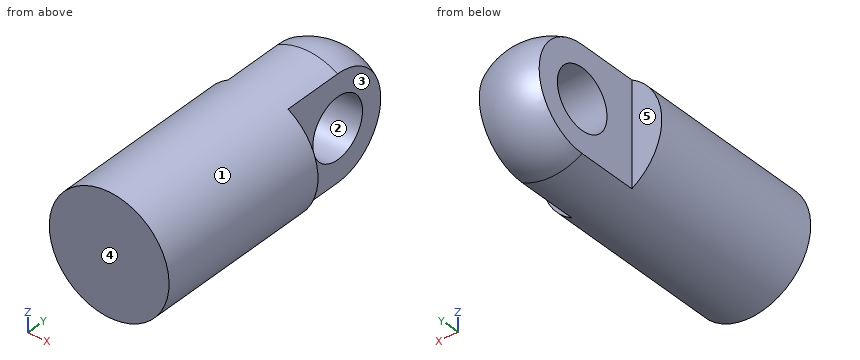
```python
from build123d import *

# Parameters (mm, degrees)
SKETCH_1_R          = 8
EXTRUDE_1_DEPTH     = 32
CUT_EXTRUDE_START   = -16
CUT_EXTRUDE_1_DEPTH = 16
SKETCH_6_R          = 4
CUT_EXTRUDE_2_DEPTH = 43.520583251


with BuildPart() as part:
    # 草图1 → 凸台-拉伸1 (new body)
    with BuildSketch(Plane(origin=(0, 0, 0), x_dir=(1, 0, 0), z_dir=(0, 1, 0))):
        with Locations(Location((0, 0, 0), (0, 0, 270))):
            Circle(SKETCH_1_R)
    extrude(amount=EXTRUDE_1_DEPTH)

    # 草图3 one side → 旋转4 (revolve)
    with BuildSketch(Plane.XY):
        with BuildLine():
            Line((0, 24), (0, 40))
            ThreePointArc((0, 40), (-8, 32), (0, 24))
        make_face()
    revolve(axis=Axis((0, 32, 0), (0, 1, 0)))

    # 草图5 → 切除-拉伸1 (cut)
    with BuildSketch(Plane(origin=(0, 40, 0), x_dir=(1, 0, 0), z_dir=(0, 1, 0)).offset(CUT_EXTRUDE_START)):
        with BuildLine():
            Line((4, -6.92820323), (4, 6.92820323))
            ThreePointArc((4, 6.92820323), (8, 0), (4, -6.92820323))
        make_face()
        with BuildLine():
            Line((-4, -6.92820323), (-4, 6.92820323))
            ThreePointArc((-4, 6.92820323), (-8, 0), (-4, -6.92820323))
        make_face()
    extrude(amount=CUT_EXTRUDE_1_DEPTH, mode=Mode.SUBTRACT)

    # 草图6 → 切除-拉伸2 (cut, through all)
    with BuildSketch(Plane(origin=(4, 0, 0), x_dir=(0, 0, -1), z_dir=(1, 0, 0))):
        with Locations((0, 32)):
            Circle(SKETCH_6_R)
    extrude(amount=-CUT_EXTRUDE_2_DEPTH, mode=Mode.SUBTRACT)


solid = part.part
```
Check sheet for the modelled part. Datum: model origin and axes. Units: mm. Face numbers are marked on the shaded views. A direction names the side the tool comes from. Round coordinates to 2 decimals unless told otherwise and drop trailing zeros. Loops run counter-clockwise (first coordinate to the right, second up) from the corner with the lowest first, then second, coordinate; pieces in that order, holes last. Notation, with made-up numbers: (-37, 68) - (-2, 68) arc R29 ccw to (-2, 100) - close; hole circle Ø6 at (16.25, 4). An arc over 180 degrees is marked (long way). Answer as a JSON object with one key per item and string values. Group by question number.
Q1. Gauge pin test, flat ends, axial feed: P1, Ø8, axis at y = 32, z = -3.5, coming from the +X side; P2, Ø1, axis at x = 2, z = -1.5, coming from the +Y side; P3, Ø1.5, axis at y = 17.5, z = 3.5, coming from the -X side; P4, Ø1.5, axis at x = 6, z = 4.5, coming from the -Y side. Record the tip position at first contact, or that the pin passes through.
Q2. Mould release check, pull along Z, two halves, no side actions. Record for the marked faces 1, 2 and 3: released by +Z, released by -Z, zero draft, split by the parting line, or undercut.
Q3. Set-up check for the marked faces 4 and 5: record each of +Z, -Z, +X, -X, +Y, -Y from which the full face is reachable in a straight line by a thin tool's end or side.
Q4. Sectioned sample at B-B, the plane y = 30.5. Enter the section's corners in (x, z).
Q5. Scan lines: line 1 along X through (y, z) = (34, -5.25); line 2 along Y through (x, z) = (-5.25, 2); line 3 along Y through (x, z) = (3, 1). Record each from-to range of solid material in increasing order. Write a range as [from, to].
Q6. Sectioned sample at A-A, the plane z = 0. Enter the section's corners in (x, y), plus the area to 3 significant figures.
Q7. Sectioned sample at C-C, the plane x = 0. Enter the section's corners in (y, z), plus the area to 3 significant figures.
Q8. Sectioned sample at D-D, the plane z = -2.25. Enter the section's corners in (x, y), plus the area to 3 significant figures.
Solution:
{
 "1": {"P1": "stops at x = 4", "P2": "stops at y = 39.75", "P3": "stops at x = -7.51", "P4": "stops at y = 0"},
 "2": {"face 1": "split by the parting line", "face 2": "undercut", "face 3": "zero draft"},
 "3": {"face 4": "+Z, -Z, +X, -X, -Y", "face 5": "+Z, -Z, -X, +Y"},
 "4": {"outline": "(-4, -6.93) arc R8 ccw to (4, -6.93) - (4, -3.71) - (-4, -3.71) - close; (-4, 3.71) - (4, 3.71) - (4, 6.93) arc R8 ccw to (-4, 6.93) - close"},
 "5": {"line 1": "x = [-4, 4]", "line 2": "y = [0, 24]", "line 3": "y = [0, 28.13], [35.87, 39.35]"},
 "6": {"outline": "(-8, 0) - (8, 0) - (8, 24) - (4, 24) - (4, 28) - (-4, 28) - (-4, 24) - (-8, 24) - close; (-4, 36) - (4, 36) - (4, 38.93) arc R8 ccw to (-4, 38.93) - close", "area": "445 mm²"},
 "7": {"outline": "(0, -8) - (32, -8) arc R8 ccw to (32, 8) - (0, 8) - close; hole circle Ø8 at (32, 0)", "area": "562 mm²"},
 "8": {"outline": "(-7.68, 0) - (7.68, 0) - (7.68, 24) - (4, 24) - (4, 28.69) - (-4, 28.69) - (-4, 24) - (-7.68, 24) - close; (-4, 35.31) - (4, 35.31) - (4, 38.55) arc R7.68 ccw to (-4, 38.55) - close", "area": "438 mm²"}
}
